from build123d import *

# Parameters (mm, degrees)
ESBO_O1_R                = 2.975
RESSALTO_EXTRUS_O1_DEPTH = 2.3
FILETE1_SIZE             = 1
FILETE1_SIZE_2           = 2
FILETE2_R                = 0.5
CORTE_EXTRUS_O1_DEPTH    = 1.3
ESBO_O3_R                = 1.45
RESSALTO_EXTRUS_O2_DEPTH = 19.8
FILETE3_R                = 0.2


with BuildPart() as part:
    # Esboço1 → Ressalto-extrusão1 (new body)
    with BuildSketch(Plane.XY):
        Circle(ESBO_O1_R)
    extrude(amount=RESSALTO_EXTRUS_O1_DEPTH)

    # Filete1
    # an asymmetric fillet: 2, 1 mm, written as the material it takes off along each edge
    with BuildSketch(Plane(origin=(0, 0, 0), x_dir=(1, 0, 0), z_dir=(0, -1, 0))) as filete1_piece_1:
        with BuildLine():
            Bezier((2.975, FILETE1_SIZE), (2.975, 0), (2.975 - FILETE1_SIZE_2, 0), weights=[1, 0.707106781, 1])
            Line((2.975 - FILETE1_SIZE_2, 0), (2.975, 0))
            Line((2.975, 0), (2.975, FILETE1_SIZE))
        make_face()
    revolve(axis=Axis((0, 0, 0), (0, 0, 1)), mode=Mode.SUBTRACT)

    # Filete2
    filete2_edges = [part.edges().sort_by_distance(p)[0] for p in [
        (-2.975, 0, 2.3),
    ]]
    fillet(filete2_edges, radius=FILETE2_R)

    # Esboço2 → Corte-extrusão1 (cut)
    with BuildSketch(Plane(origin=(0, 0, 0), x_dir=(-1, 0, 0), z_dir=(0, 0, -1))):
        with BuildLine():
            Line((0.25, -2.25), (-0.25, -2.25))
            ThreePointArc((-0.25, -2.25), (-0.356066017, -2.206066017), (-0.4, -2.1))
            Line((-0.4, -2.1), (-0.4, -0.7))
            ThreePointArc((-0.4, -0.7), (-0.487867966, -0.487867966), (-0.7, -0.4))
            Line((-0.7, -0.4), (-2.1, -0.4))
            ThreePointArc((-2.1, -0.4), (-2.206066017, -0.356066017), (-2.25, -0.25))
            Line((-2.25, -0.25), (-2.25, 0.25))
            ThreePointArc((-2.25, 0.25), (-2.206066017, 0.356066017), (-2.1, 0.4))
            Line((-2.1, 0.4), (-0.7, 0.4))
            ThreePointArc((-0.7, 0.4), (-0.487867966, 0.487867966), (-0.4, 0.7))
            Line((-0.4, 0.7), (-0.4, 2.1))
            ThreePointArc((-0.4, 2.1), (-0.356066017, 2.206066017), (-0.25, 2.25))
            Line((-0.25, 2.25), (0.25, 2.25))
            ThreePointArc((0.25, 2.25), (0.356066017, 2.206066017), (0.4, 2.1))
            Line((0.4, 2.1), (0.4, 0.7))
            ThreePointArc((0.4, 0.7), (0.487867966, 0.487867966), (0.7, 0.4))
            Line((0.7, 0.4), (2.1, 0.4))
            ThreePointArc((2.1, 0.4), (2.206066017, 0.356066017), (2.25, 0.25))
            Line((2.25, 0.25), (2.25, -0.25))
            ThreePointArc((2.25, -0.25), (2.206066017, -0.356066017), (2.1, -0.4))
            Line((2.1, -0.4), (0.7, -0.4))
            ThreePointArc((0.7, -0.4), (0.487867966, -0.487867966), (0.4, -0.7))
            Line((0.4, -0.7), (0.4, -2.1))
            ThreePointArc((0.4, -2.1), (0.356066017, -2.206066017), (0.25, -2.25))
        make_face()
    extrude(amount=-CORTE_EXTRUS_O1_DEPTH, mode=Mode.SUBTRACT)

    # Esboço3 → Ressalto-extrusão2 (add)
    with BuildSketch(Plane.XY.offset(2.3)):
        with Locations(Location((0, 0, 0), (0, 0, 180))):
            Circle(ESBO_O3_R)
    extrude(amount=RESSALTO_EXTRUS_O2_DEPTH)

    # Filete3
    filete3_edges = [part.edges().sort_by_distance(p)[0] for p in [
        (1.45, 0, 22.1),
    ]]
    fillet(filete3_edges, radius=FILETE3_R)


solid = part.part
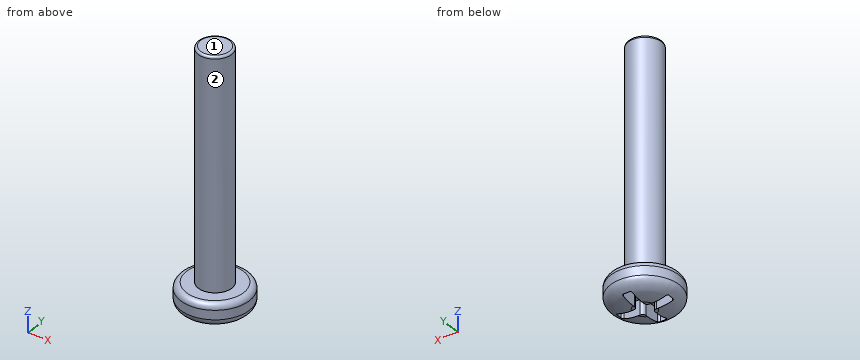
CAD build for the part. Positions are in the model's coordinates, mm. Face numbers are marked on the shaded views. A direction names the side the tool comes from. Round coordinates to 2 decimals unless told otherwise and drop trailing zeros. Write each loop counter-clockwise with the first axis right and the second up, starting at its lowest first coordinate (ties: lowest second). Pieces come first, ordered by that corner, then holes. Notation, with made-up numbers: M 49,-26.5 L 85,-26.5 A18 cw 85,7.5 Z; hole C -25.5,52.25 d4. An arc over 180 degrees is marked long. Use a Markdown table: item, result. Add a question column.
1. 3-axis set-ups, long thin cutter, end or side, ignore diameter. For the marked faces 1 and 2: which of +Z, -Z, +X, -X, +Y, -Y reach the whole face in a straight line?
2. Slice it at A-A on z = 9. Give the cut face in (x, y).
3. Drill centre lines: probe 1 along Z at (x, y) = (0.5, 0); probe 2 along Z at (x, y) = (-0.05, -1.5); probe 3 along Y at (x, z) = (1.05, 3.75). Where is each one in solid material? Low to high.
4. Slice it at B-B on z = 1.5. Give the cut face in (x, y) (3 decimals), then the cut area to 3 significant figures.
5. Flat gauge pins, fed straight in: P1, Ø1, axis at x = 1, z = 1, coming from the -Y side; P2, Ø0.7, axis at y = -1.5, z = 1, coming from the +X side; P3, Ø0.7, axis at y = -1.5, z = 1, coming from the -X side. Where does each tip first touch, or does it go through?
Reply:
| question | item | result |
|---|---|---|
| 1 | face 1 | +Z, +X, -X, +Y, -Y |
| 1 | face 2 | +Z |
| 2 | outline | C 0,0 d2.9 |
| 3 | probe 1 | z = 1.3 to 22.1 |
| 3 | probe 2 | z = 1.3 to 2.3 |
| 3 | probe 3 | y = -1 to 1 |
| 4 | outline | C 0,0 d5.95 |
| 4 | area | 27.8 mm^2 |
| 5 | P1 | stops at y = -2.93 |
| 5 | P2 | stops at x = 2.74 |
| 5 | P3 | stops at x = -2.74 |
